Could you check a few things on this model? Use its own coordinates, in mm. Coordinates: 2 decimals unless noted, no trailing zeros. Order: outer loops, then holes, each group sorted by start corner. A loop starts at its lowest first (then second) coordinate and runs counter-clockwise, first axis right, second up. Notation, with made-up numbers: (38, 18) - (48, 18) arc R9 ccw to (48, 35) - close; hole circle Ø8 at (47, 74.5). An arc over 180 degrees is marked (long way). One line per item, written item: value. Start each with the question number.
from build123d import *

# Parameters (mm, degrees)
F0_W        = 200
F0_H        = 40
F0_R        = 15
F1_DEPTH    = 30
F2_T1_DEPTH = 160
F2_T3_DEPTH = 300


# Not quite as in the source:
# - a fillet or chamfer that OpenCascade refuses, or shapes differently, is made with other operations: its cross-section is extruded or revolved along the edge and cut away or added


with BuildPart() as f1:
    # F0 (on Front) → F1 (new body, symmetric)
    with BuildSketch(Plane.XZ):
        with Locations((-100, -20)):
            Rectangle(F0_W, F0_H)
        with Locations((-100, -20)):
            Circle(F0_R, mode=Mode.SUBTRACT)
    extrude(amount=F1_DEPTH, both=True)

    # F2: fillet of radius 20 on 4 edges, made by hand

    # F2_s2 → F2_t1 (cut)
    with BuildSketch(Plane.XZ.offset(-80)):
        with BuildLine():
            ThreePointArc((-180, 0), (-194.1421356237, -5.8578643763), (-200, -20))
            Line((-200, -20), (-200, 0))
            Line((-200, 0), (-180, 0))
        make_face()
        with BuildLine():
            ThreePointArc((0, -20), (-5.8578643763, -34.1421356237), (-20, -40))
            Line((-20, -40), (0, -40))
            Line((0, -40), (0, -20))
        make_face()
    extrude(amount=F2_T1_DEPTH, mode=Mode.SUBTRACT)

    # F2_s4 → F2_t3 (cut)
    with BuildSketch(Plane.YZ.offset(-250)):
        with BuildLine():
            ThreePointArc((-10, 0), (-24.1421356237, -5.8578643763), (-30, -20))
            Line((-30, -20), (-30, 0))
            Line((-30, 0), (-10, 0))
        make_face()
        with BuildLine():
            ThreePointArc((10, -40), (24.1421356237, -34.1421356237), (30, -20))
            Line((30, -20), (30, -40))
            Line((30, -40), (10, -40))
        make_face()
    extrude(amount=F2_T3_DEPTH, mode=Mode.SUBTRACT)


solid = f1.part
Q1. I want a section at A-A on z = -32. Please give me the cut outline in (x, y), then the cut area to 3 significant figures.
Q2. I want a section at D-D on x = -38. Please give me the cut outline in (y, z).
Q3. I want a section at C-C on x = -100. Please give me the cut outline in (y, z).
Q4. I'm going to push flat-ended pins straight in: pin 1 (1 mm diameter, centred on y = 5, z = -13.5, fed in from -X); pin 2 (12 mm diameter, centred on y = -19, z = -32.5, fed in from +X); pin 3 (1.5 mm diameter, centred on x = -128.5, y = 17.5, fed in from -Z). Where does each tip first touch, or does it pass through?
Q5. I want a section at B-B on y = -2.5. Please give me the cut outline in (x, z), then the cut area to 3 significant figures.
Q6. If I drill on L1, parallel to Z at x = -100, y = 2; L2, parallel to Y at x = -17, z = -21; L3, parallel to X at y = -3, z = -29, over which ranges is the centre line in solid material (lowest first)?
Q7. We'd pull the mould along Z, two halves only. Please class faces 1 (the cylindrical face through (-114.985, 0.42, -19.34)), 2 (the flat face through (-101, 30, -3)), 3 (the flat face through (-111, -10, -40)), 4 (the flat face through (-91, 10, 0)): +Z half, -Z half, draft (parallel to the pull), parting line (faces both ways), or undercut.
Values follow:
1. outline: (-200, -30) - (-109, -30) - (-109, 26) - (-200, 26) - close; (-91, -30) - (-4, -30) - (-4, 26) - (-91, 26) - close
1. area: 9,970 mm^2
2. outline: (-30, -40) - (10, -40) arc R20 ccw to (30, -20) - (30, 0) - (-10, 0) arc R20 ccw to (-30, -20) - close
3. outline: (-30, -40) - (10, -40) arc R20 ccw to (23.23, -35) - (-30, -35) - close; (-23.23, -5) - (30, -5) - (30, 0) - (-10, 0) arc R20 ccw to start
4. pin 1: stops at x = -199.08
4. pin 2: stops at x = -1.09
4. pin 3: stops at z = -38.83
5. outline: (-200, -40) - (-20, -40) arc R20 ccw to (0, -20) - (0, 0) - (-180, 0) arc R20 ccw to (-200, -20) - close; hole circle Ø30 at (-100, -20)
5. area: 7,120 mm^2
6. L1: z = -40 to -35, -5 to 0
6. L2: y = -30 to 29.97
6. L3: x = -200 to -112, -88 to -2.14
7. face 1: undercut
7. face 2: draft
7. face 3: -Z half
7. face 4: +Z half
